Part print with two shaded views. Sizes in mm from the minimum x, y, z corner. A direction names the side the tool comes from. Round coordinates to 2 decimals unless told otherwise and drop trailing zeros. Write each loop counter-clockwise with the first axis right and the second up, starting at its lowest first coordinate (ties: lowest second). Pieces come first, ordered by that corner, then holes. Notation, with made-up numbers: (4.25, 42) -> (43.25, 42) arc R19 ccw to (43.25, 68) -> close; hole circle Ø11 at (9.25, 9.25). An arc over 180 degrees is marked (long way). Answer in a Markdown table with one row per item.
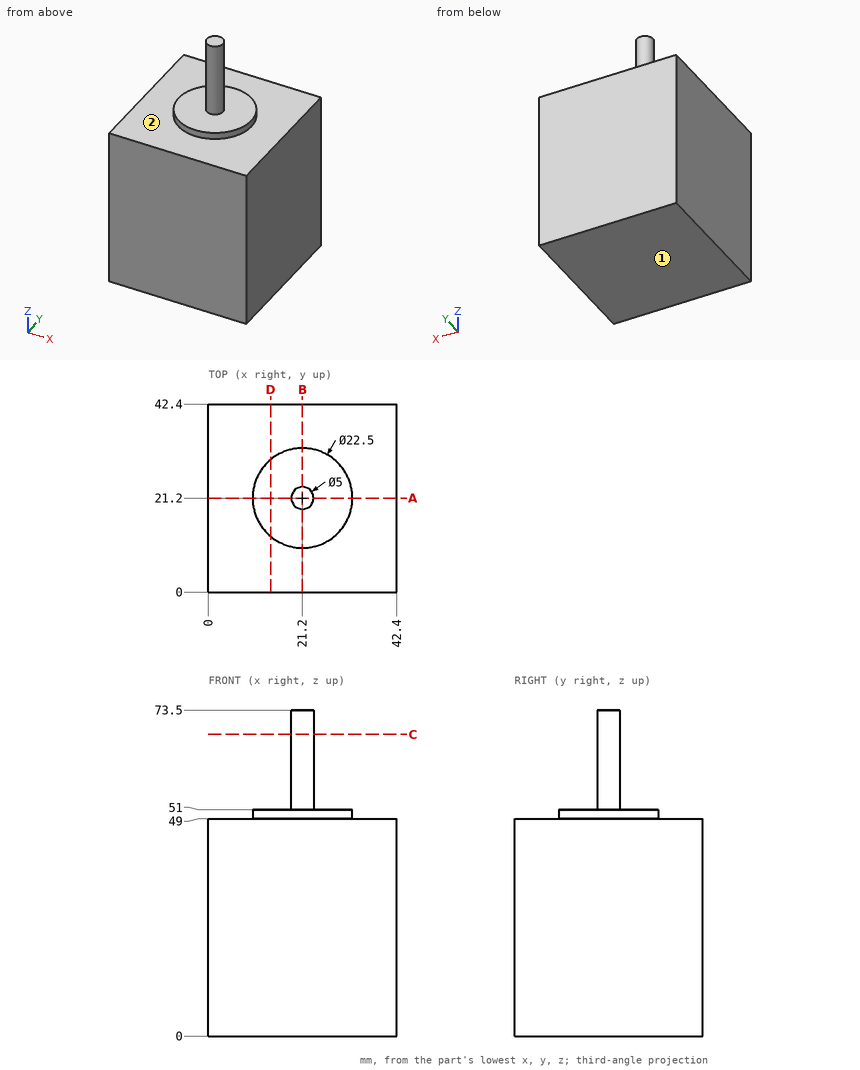
Q1. Saw through at C-C on z = 68. Write the cut outline in (x, y), plus the area to 3 significant figures.
A:
| item | result |
|---|---|
| outline | circle Ø5 at (21.2, 21.2) |
| area | 19.6 mm² |
Q2. Saw through at D-D on x = 14. Write the cut outline in (y, z), plus the area to 3 significant figures.
A:
| item | result |
|---|---|
| outline | (0, 0) -> (42.4, 0) -> (42.4, 49) -> (29.84, 49) -> (29.84, 51) -> (12.56, 51) -> (12.56, 49) -> (0, 49) -> close |
| area | 2,110 mm² |
Q3. Wall check: line 1 (X direction, y = 21.5, z = 58); line 2 (Z direction, x = 32.5, y = 13.5); line 3 (Z direction, x = 27.5, y = 12). Give the ranges that are in metal, low to high. Write a range as [from, to].
A:
| item | result |
|---|---|
| line 1 | [18.72, 23.68] |
| line 2 | [0, 49] |
| line 3 | [0, 51] |
Q4. Saw through at A-A on y = 21.2. Write the cut outline in (x, z).
A:
| item | result |
|---|---|
| outline | (0, 0) -> (42.4, 0) -> (42.4, 49) -> (32.45, 49) -> (32.45, 51) -> (23.7, 51) -> (23.7, 73.5) -> (18.7, 73.5) -> (18.7, 51) -> (9.95, 51) -> (9.95, 49) -> (0, 49) -> close |
Q5. Drop flat-ended pins along their axis: P1, Ø10, axis at x = 16, z = 61.5, coming from the -Y side; P2, Ø2, axis at x = 25.5, y = 8.5, coming from the +Z side. Give the stop position or say it passes through.
A:
| item | result |
|---|---|
| P1 | y = 18.71 |
| P2 | z = 49 |
Q6. Which spindle directions (+Z, -Z, +X, -X, +Y, -Y) get a long thin tool onto all of the face, cutting with end or side? Do the marked faces 1 and 2. Say none if no direction does.
A:
| item | result |
|---|---|
| face 1 | -Z, +X, -X, +Y, -Y |
| face 2 | +Z |
